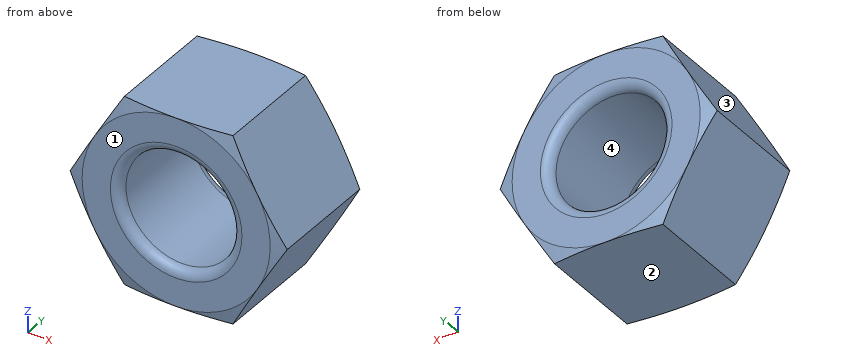
from build123d import *

# Parameters (mm, degrees)
F0_R     = 12
F1_DEPTH = 25
F4_R     = 2


with BuildPart() as f1:
    # F0 (on Front) → F1 (new body)
    with BuildSketch(Plane.XZ):
        Polygon((11.547005, 20), (-11.547005, 20), (-23.094011, 0), (-11.547005, -20), (11.547005, -20), (23.094011, 0), align=None)
        Circle(F0_R, mode=Mode.SUBTRACT)
    extrude(amount=F1_DEPTH)

    # F2 (on Right) → F3 (revolve, cut)
    with BuildSketch(Plane.YZ):
        Polygon((-25, 56.939398), (-25, 20), (-18.841215, 42.984898), (-6.158785, 42.984898), (0, 20), (0, 56.939398), align=None)
    revolve(axis=Axis((0, -3.116442, 0), (0, 1, 0)), mode=Mode.SUBTRACT)

    # F4
    f4_edges = [f1.edges().sort_by_distance(p)[0] for p in [
        (-12, -25, 0),
        (-12, 0, 0),
    ]]
    fillet(f4_edges, radius=F4_R)


solid = f1.part
Part model, mm, in its own coordinate system. Face numbers are marked on the shaded views. Coordinates: 2 decimals unless noted, no trailing zeros. Order: outer loops, then holes, each group sorted by start corner. A loop starts at its lowest first (then second) coordinate and runs counter-clockwise, first axis right, second up. Notation, with made-up numbers: M 66.5,4 L 76.5,4 A24 ccw 76.5,30 Z; hole C 55.5,-7 d1. An arc over 180 degrees is marked long. Use a Markdown table: item, result.
(1) Pull direction Z, two halves, no side cores. Call the marked faces 1, 2, 3 and 4: released by +Z, released by -Z, zero draft, split by the parting line, or undercut.
A:
| item | result |
|---|---|
| face 1 | zero draft |
| face 2 | released by -Z |
| face 3 | released by +Z |
| face 4 | undercut |
(2) Flat gauge pins, fed straight in: pin 1 (10 mm diameter, centred on y = -12, z = 0.5, fed in from +X); pin 2 (5 mm diameter, centred on y = -7, z = 10.5, fed in from +X); pin 3 (4 mm diameter, centred on y = -16.5, z = 3, fed in from +X). Where does each tip first touch, or does it go through?
A:
| item | result |
|---|---|
| pin 1 | stops at x = 23.09 |
| pin 2 | stops at x = 18.48 |
| pin 3 | stops at x = 22.52 |
(3) Cut at A-A on y = -9. Write the cut outline in (x, z), then the cut area to 3 significant figures.
A:
| item | result |
|---|---|
| outline | M -23.09,0 L -11.55,-20 L 11.55,-20 L 23.09,0 L 11.55,20 L -11.55,20 Z; hole C 0,0 d24 |
| area | 933 mm^2 |
(4) Probe L1, parallel to Z at x = 0, y = -10.5; L2, parallel to X at y = -15.5, z = 0.5; L3, parallel to Z at x = -7.5, y = -14.75. List the from-to ranges inside material, lowest first.
A:
| item | result |
|---|---|
| L1 | z = -20 to -12, 12 to 20 |
| L2 | x = -22.81 to -11.99, 11.99 to 22.81 |
| L3 | z = -20 to -9.37, 9.37 to 20 |
